Geometry: final body of the model. Coordinates: model frame, mm. Face numbers are marked on the shaded views. A direction names the side the tool comes from. Coordinates: 2 decimals unless noted, no trailing zeros. Loops run counter-clockwise (first coordinate to the right, second up) from the corner with the lowest first, then second, coordinate; pieces in that order, holes last. Notation, with made-up numbers: (72.5, 27) -> (114.5, 27) arc R17 cw to (114.5, 32) -> close; hole circle Ø11 at (25, -32). An arc over 180 degrees is marked (long way). One line per item, written item: value. Start each with the question number.
Item 1: Mould query, pull axis X, two halves, no side actions, for the marked faces 3, 4 and 5. Classes: +X half, -X half, draft (parallel to the pull), parting line (faces both ways), or undercut.
Item 2: Ray query, probe 1 along Z at (x, y) = (-1, -11); probe 2 along Y at (x, z) = (19, 7); probe 3 along Y at (x, z) = (-6.5, 0.5). Return the intervals inside material, ascending. Write a range as from..to.
Item 3: Set-up query: the marked faces 1 and 2. Return all of +Z, -Z, +X, -X, +Y, -Y with unobstructed straight access to the full face (end or side cutting, diameter ignored); none if empty.
Item 4: Section query D-D on y = -4.9. Return loops of the section in (x, z).
Item 5: Contact query for flat-ended pins moving along their axis: pin 1 Ø1.5 at (y, z) = (-5, 6.5) entering from -X; pin 2 Ø3 at (x, z) = (-22.5, 4.5) entering from -Y; pin 3 Ø9 at (x, y) = (0, 9.8) entering from +Z; pin 4 Ø8 at (x, y) = (-8.49, -4.9) entering from -Z. Output: stop coordinate, or through.
Item 6: Section query C-C on y = 9.8. Return loops of the section in (x, z).
Item 7: Section query B-B on z = 4.5. Return loops of the section in (x, y).
Item 8: Section query A-A on x = 0. Return loops of the section in (y, z), then the cut area to 4 significant figures.
from build123d import *

# Parameters (mm, degrees)
SKETCH_1_R          = 35
EXTRUDE_1_DEPTH     = 10
CUT_EXTRUDE_1_DEPTH = 8
SKETCH_4_R          = 3.5
CUT_EXTRUDE_2_DEPTH = 1.5
SKETCH_6_R          = 2
CUT_EXTRUDE_3_DEPTH = 51.222007128


with BuildPart() as part:
    # 草图1 → 凸台-拉伸1 (new body)
    with BuildSketch(Plane.XY):
        Circle(SKETCH_1_R)
    extrude(amount=EXTRUDE_1_DEPTH)

    # 草图2 → 切除-拉伸1 (cut)
    with BuildSketch(Plane.XY.offset(10)):
        with BuildLine():
            ThreePointArc((21.428660714, 1.75), (0, 21.5), (-21.428660714, 1.75))
            Line((-21.428660714, 1.75), (-24.9, 1.75))
            Line((-24.9, 1.75), (-24.9, -1.75))
            Line((-24.9, -1.75), (-21.428660714, -1.75))
            ThreePointArc((-21.428660714, -1.75), (0, -21.5), (21.428660714, -1.75))
            Line((21.428660714, -1.75), (24.9, -1.75))
            Line((24.9, -1.75), (24.9, 1.75))
            Line((24.9, 1.75), (21.428660714, 1.75))
        make_face()
    extrude(amount=-CUT_EXTRUDE_1_DEPTH, mode=Mode.SUBTRACT)

    # 草图4 → 切除-拉伸2 (cut)
    with BuildSketch(Plane(origin=(0, 0, 0), x_dir=(-1, 0, 0), z_dir=(0, 0, -1))):
        with Locations((8.487048957, -4.9)):
            Circle(SKETCH_4_R)
        with Locations((-8.487048957, -4.9)):
            Circle(SKETCH_4_R)
        with Locations((0, 9.8)):
            Circle(SKETCH_4_R)
    extrude(amount=-CUT_EXTRUDE_2_DEPTH, mode=Mode.SUBTRACT)

    # 草图6 → 切除-拉伸3 (cut, through all)
    with BuildSketch(Plane(origin=(0, 0, 1.5), x_dir=(-1, 0, 0), z_dir=(0, 0, -1))):
        with Locations((0, 9.8)):
            Circle(SKETCH_6_R)
        with Locations((8.487048957, -4.9)):
            Circle(SKETCH_6_R)
        with Locations((-8.487048957, -4.9)):
            Circle(SKETCH_6_R)
    extrude(amount=-CUT_EXTRUDE_3_DEPTH, mode=Mode.SUBTRACT)


solid = part.part
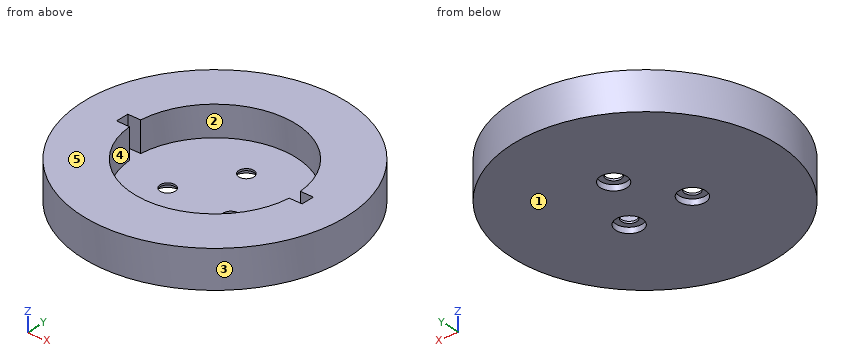
Reply:
1. face 3: parting line
1. face 4: undercut
1. face 5: draft
2. probe 1: z = 0..2
2. probe 2: y = -29.39..-10.06, 10.06..29.39
2. probe 3: y = -34.39..-7.78, -2.02..34.39
3. face 1: -Z, +X, -X, +Y, -Y
3. face 2: +Z
4. outline: (-34.66, 0) -> (-11.99, 0) -> (-11.99, 1.5) -> (-10.49, 1.5) -> (-10.49, 2) -> (-20.93, 2) -> (-20.93, 10) -> (-34.66, 10) -> close; (-6.49, 1.5) -> (-4.99, 1.5) -> (-4.99, 0) -> (4.99, 0) -> (4.99, 1.5) -> (6.49, 1.5) -> (6.49, 2) -> (-6.49, 2) -> close; (10.49, 1.5) -> (11.99, 1.5) -> (11.99, 0) -> (34.66, 0) -> (34.66, 10) -> (20.93, 10) -> (20.93, 2) -> (10.49, 2) -> close
5. pin 1: stops at x = -34.74
5. pin 2: stops at y = -28
5. pin 3: stops at z = 2
5. pin 4: stops at z = 0
6. outline: (-33.6, 0) -> (-3.5, 0) -> (-3.5, 1.5) -> (-2, 1.5) -> (-2, 2) -> (-19.14, 2) -> (-19.14, 10) -> (-33.6, 10) -> close; (2, 1.5) -> (3.5, 1.5) -> (3.5, 0) -> (33.6, 0) -> (33.6, 10) -> (19.14, 10) -> (19.14, 2) -> (2, 2) -> close
7. outline: circle Ø70 at (0, 0); hole (-24.9, -1.75) -> (-21.43, -1.75) arc R21.5 ccw to (21.43, -1.75) -> (24.9, -1.75) -> (24.9, 1.75) -> (21.43, 1.75) arc R21.5 ccw to (-21.43, 1.75) -> (-24.9, 1.75) -> close
8. outline: (-35, 0) -> (6.3, 0) -> (6.3, 1.5) -> (7.8, 1.5) -> (7.8, 2) -> (-21.5, 2) -> (-21.5, 10) -> (-35, 10) -> close; (11.8, 1.5) -> (13.3, 1.5) -> (13.3, 0) -> (35, 0) -> (35, 10) -> (21.5, 10) -> (21.5, 2) -> (11.8, 2) -> close
8. area: 343.5 mm²
